```python
from build123d import *

# Parameters (mm, degrees)
ESQUISSE1_W             = 200
ESQUISSE1_H             = 200
BOSS_EXTRU_1_DEPTH      = 250
ESQUISSE2_R             = 70
ENL_V_MAT_EXTRU_1_DEPTH = 10
ESQUISSE3_R             = 70
BOSS_EXTRU_2_DEPTH      = 10


with BuildPart() as part:
    # Esquisse1 → Boss.-Extru.1 (new body)
    with BuildSketch(Plane.XY):
        with Locations((-100, -100)):
            Rectangle(ESQUISSE1_W, ESQUISSE1_H)
    extrude(amount=BOSS_EXTRU_1_DEPTH)

    # Esquisse2 → Enlèv. mat.-Extru.1 (cut)
    with BuildSketch(Plane(origin=(0, 0, 0), x_dir=(-1, 0, 0), z_dir=(0, 0, -1))):
        with Locations((100, -100)):
            Circle(ESQUISSE2_R)
    extrude(amount=-ENL_V_MAT_EXTRU_1_DEPTH, mode=Mode.SUBTRACT)

    # Esquisse3 → Boss.-Extru.2 (add)
    with BuildSketch(Plane(origin=(0, 0, 0), x_dir=(0, 0, -1), z_dir=(1, 0, 0))):
        with Locations(Location((-125, -100, 0), (0, 0, 90))):
            Circle(ESQUISSE3_R)
    extrude(amount=BOSS_EXTRU_2_DEPTH)


solid = part.part
```
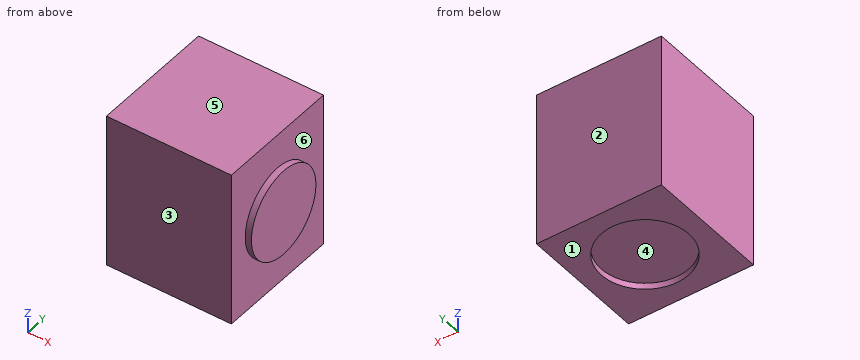
For this review, take the finished solid that the model builds, in its own axes (mm). Face numbers are marked on the shaded views. A direction names the side the tool comes from. Round coordinates to 2 decimals unless told otherwise and drop trailing zeros. Write each loop counter-clockwise with the first axis right and the second up, starting at its lowest first coordinate (ties: lowest second). Pieces come first, ordered by that corner, then holes. Notation, with made-up numbers: (83.5, -21.75) - (122.5, -21.75) arc R20 ccw to (122.5, 15.25) - close; hole circle Ø7 at (13.5, -38). An arc over 180 degrees is marked (long way). Answer as CSV lines item,"result". Start each with the question number.
(1) Machinability: for the marked faces 5 and 6, which of the approach directions +Z, -Z, +X, -X, +Y, -Y give a long, thin tool a straight path to every point of the face, cutting with its end or side? Answer none if there is none.
(2) Add section A-A, the plane x = -100. State the section outline as (y, z) points, plus the area to 3 significant figures.
(3) Add section C-C, the plane z = 191. State the section outline as (x, y) points, plus the area to 3 significant figures.
(4) For line 1 (Y direction, x = -100, z = 7); line 2 (X direction, y = -59, z = 65); line 3 (Z direction, x = -166.5, y = -93), list the stretches that pass through material, from the lowest coordinate up.
(5) Add section B-B, the plane y = -26. State the section outline as (x, z) points, plus the area to 3 significant figures.
(6) For pin 1 (10 mm diameter, centred on x = -121.5, y = -160.5, fed in from -Z), flat-tipped, find the tip position at first contact; note if it passes through.
(7) Mouldability with a two-part tool opening along Y and no side actions: class the marked faces 1, 2, 3 and 4 as +Y half, -Y half, draft (parallel to the pull), parting line (faces both ways), or undercut.
(8) Add section D-D, the plane z = 229. State the section outline as (x, y) points.
From the geometry:
1,face 5,"+Z, +X, -X, +Y, -Y"
1,face 6,"+X"
2,outline,"(-200, 0) - (-170, 0) - (-170, 10) - (-30, 10) - (-30, 0) - (0, 0) - (0, 250) - (-200, 250) - close"
2,area,"48,600 mm²"
3,outline,"(-200, -200) - (0, -200) - (0, -123.32) - (10, -123.32) - (10, -76.68) - (0, -76.68) - (0, 0) - (-200, 0) - close"
3,area,"40,500 mm²"
4,line 1,"y = -200 to -170, -30 to 0"
4,line 2,"x = -200 to 0"
4,line 3,"z = 10 to 250"
5,outline,"(-200, 0) - (0, 0) - (0, 250) - (-200, 250) - close"
5,area,"50,000 mm²"
6,pin 1,"stops at z = 10"
7,face 1,"draft"
7,face 2,"+Y half"
7,face 3,"-Y half"
7,face 4,"undercut"
8,outline,"(-200, -200) - (0, -200) - (0, 0) - (-200, 0) - close"
